The model under review builds one solid part; all positions refer to its coordinate system, in mm. A direction names the side the tool comes from. Coordinates: 2 decimals unless noted, no trailing zeros. Loops run counter-clockwise (first coordinate to the right, second up) from the corner with the lowest first, then second, coordinate; pieces in that order, holes last. Notation, with made-up numbers: (37, -33.75) - (85, -33.75) arc R30 ccw to (85, -2.75) - close; hole circle Ø6 at (0, 84.5). An arc over 180 degrees is marked (long way). Answer in a Markdown table with one row per item. Add a question column.
(1) We need section C-C on y = 18. Write out the cut boundary in (x, z).
(2) We need section A-A on z = 0.4. Write out the cut boundary in (x, y).
(3) Mouldability with a two-part tool opening along X and no side actions: class faces 3 (the flat face through (64, 49, 2)), 4 (the cylindrical face through (2.85, 3.01, 1.01)) as +X half, -X half, draft (parallel to the pull), parting line (faces both ways), or undercut.
(4) Machinability: for faces 1 (the cylindrical face through (122.99, 2.85, 1.01)), 2 (the flat face through (64, 49, 0)), which of the approach directions +Z, -Z, +X, -X, +Y, -Y give a long, thin tool a straight path to every point of the face, cutting with its end or side? Answer none if there is none.
(5) We need section B-B on x = 44. Write out the cut boundary in (y, z), plus the area to 3 significant figures.
(6) For P1, Ø5, axis at x = 55.5, y = 48.5, coming from the -Z side, flat-tipped, find the tip position at first contact; note if it passes through.
(7) For line 1 along X through (y, z) = (11, 1.25); line 2 along Y through (x, z) = (114, 1.65); line 3 along Y through (x, z) = (119.5, 1.75), list the stretches that pass through material, from the lowest coordinate up.
from build123d import *

# Parameters (mm, degrees)
BOX003_W     = 126
BOX003_H     = 46
BOX003_DEPTH = 10
FILLET005_R  = 10
BOX004_W     = 150
BOX004_H     = 70
BOX004_DEPTH = 2


with BuildPart() as fillet005:
    # Box003 → Box003 (new body)
    with BuildSketch(Plane.XY):
        with Locations((63, 23)):
            Rectangle(BOX003_W, BOX003_H)
    extrude(amount=BOX003_DEPTH)

    # Fillet005
    fillet005_edges = [fillet005.edges().sort_by_distance(p)[0] for p in [
        (0, 0, 5),
        (0, 46, 5),
        (126, 0, 5),
        (126, 46, 5),
    ]]
    fillet(fillet005_edges, radius=FILLET005_R)


with BuildPart() as cut001:
    # Box004 → Box004 (new body)
    with BuildSketch(Plane(origin=(-10, -10, 0), x_dir=(1, 0, 0), z_dir=(0, 0, 1))):
        with Locations((75, 35)):
            Rectangle(BOX004_W, BOX004_H)
    extrude(amount=BOX004_DEPTH)

    # Cut001: cut Fillet005
    add(fillet005.part, mode=Mode.SUBTRACT)


solid = cut001.part
Outcome:
| question | item | result |
|---|---|---|
| 1 | outline | (-10, 0) - (0, 0) - (0, 2) - (-10, 2) - close; (126, 0) - (140, 0) - (140, 2) - (126, 2) - close |
| 2 | outline | (-10, -10) - (140, -10) - (140, 60) - (-10, 60) - close; hole (0, 10) arc R10 ccw to (10, 0) - (116, 0) arc R10 ccw to (126, 10) - (126, 36) arc R10 ccw to (116, 46) - (10, 46) arc R10 ccw to (0, 36) - close |
| 3 | face 3 | draft |
| 3 | face 4 | undercut |
| 4 | face 1 | +Z, -Z |
| 4 | face 2 | -Z, +X, -X, +Y, -Y |
| 5 | outline | (-10, 0) - (0, 0) - (0, 2) - (-10, 2) - close; (46, 0) - (60, 0) - (60, 2) - (46, 2) - close |
| 5 | area | 48.0 mm² |
| 6 | P1 | z = 0 |
| 7 | line 1 | -10 to 0, 126 to 140 |
| 7 | line 2 | -10 to 0, 46 to 60 |
| 7 | line 3 | -10 to 0.63, 45.37 to 60 |
